from build123d import *

# Parameters (mm, degrees)
F0_R     = 15.875
F0_R_2   = 1.5875
F0_R_3   = 7.9375
F1_DEPTH = 1.5875


with BuildPart() as f1:
    # F0 (on Top) → F1 (new body, symmetric)
    with BuildSketch(Plane.XY):
        Circle(F0_R)
        with Locations((0, -12.7)):
            Circle(F0_R_2, mode=Mode.SUBTRACT)
        with Locations((-12.7, 0)):
            Circle(F0_R_2, mode=Mode.SUBTRACT)
        Circle(F0_R_3, mode=Mode.SUBTRACT)
        with Locations((12.7, 0)):
            Circle(F0_R_2, mode=Mode.SUBTRACT)
        with Locations((0, 12.7)):
            Circle(F0_R_2, mode=Mode.SUBTRACT)
    extrude(amount=F1_DEPTH, both=True)


solid = f1.part
Design review of the part built by this model. Coordinates are the model's own, in mm. Coordinates: 2 decimals unless noted, no trailing zeros. Order: outer loops, then holes, each group sorted by start corner. A loop starts at its lowest first (then second) coordinate and runs counter-clockwise, first axis right, second up.
Item 1: Take a section at D-D, the plane y = -4. Write out the cut boundary in (x, z).
Item 2: The part is to be moulded in two halves that separate along Y. For faces 1 (the cylindrical face through (-11.186, 0.477, -0.022)), 2 (the cylindrical face through (-3.441, -15.497, 0.022)), 3 (the flat face through (-3.8, 7.3, 1.588)), say which applies: pulls with the +Y half, pulls with the -Y half, needs draft (parallel to the pull), parting line crosses it, or undercut.
Item 3: Take a section at A-A, the plane x = 6. Write out the cut boundary in (y, z), then the cut area to 3 significant figures.
Item 4: Take a section at C-C, the plane x = 1. Write out the cut boundary in (y, z).
Item 5: For line 1 (Y direction, x = 0, z = 0.6) (1 decimal); line 2 (X direction, y = 1, z = 0); line 3 (Y direction, x = -14, z = -1.35), list the stretches that pass through material, from the lowest coordinate up.
Item 6: For pin 1 Ø1.5 at (x, y) = (6.5, 1.5) entering from -Z; pin 2 Ø1.5 at (y, z) = (-5.5, 1) entering from +X; pin 3 Ø1 at (y, z) = (9, -0.5) entering from +X, all flat-tipped, find the tip position at first contact; note any pin that passes through.
Item 7: Take a section at B-B, the plane z = -0.05. Count the separate pieces of the cut face and the enclosed holes in it, then the cut area to 3 significant figures.
The answers:
1. outline: (-15.36, -1.59) - (-6.86, -1.59) - (-6.86, 1.59) - (-15.36, 1.59) - close; (6.86, -1.59) - (15.36, -1.59) - (15.36, 1.59) - (6.86, 1.59) - close
2. face 1: undercut
2. face 2: parting line crosses it
2. face 3: needs draft
3. outline: (-14.7, -1.59) - (-5.2, -1.59) - (-5.2, 1.59) - (-14.7, 1.59) - close; (5.2, -1.59) - (14.7, -1.59) - (14.7, 1.59) - (5.2, 1.59) - close
3. area: 60.3 mm2
4. outline: (-15.84, -1.59) - (-13.93, -1.59) - (-13.93, 1.59) - (-15.84, 1.59) - close; (-11.47, -1.59) - (-7.87, -1.59) - (-7.87, 1.59) - (-11.47, 1.59) - close; (7.87, -1.59) - (11.47, -1.59) - (11.47, 1.59) - (7.87, 1.59) - close; (13.93, -1.59) - (15.84, -1.59) - (15.84, 1.59) - (13.93, 1.59) - close
5. line 1: y = -15.9 to -14.3, -11.1 to -7.9, 7.9 to 11.1, 14.3 to 15.9
5. line 2: x = -15.84 to -13.93, -11.47 to -7.87, 7.87 to 11.47, 13.93 to 15.84
5. line 3: y = -7.48 to -0.91, 0.91 to 7.48
6. pin 1: passes through
6. pin 2: stops at x = 15.15
6. pin 3: stops at x = 13.41
7. separate pieces: 1
7. enclosed holes: 5
7. area: 562 mm2
